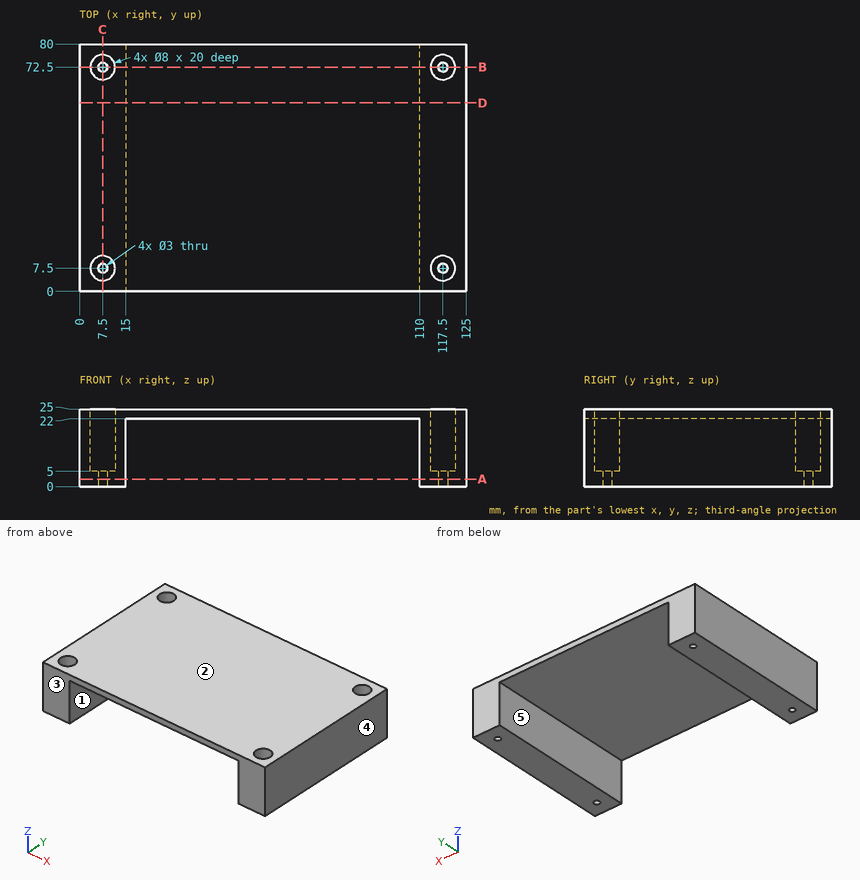
The figure shows three views and two pictorial views of one solid part (mm, origin at its lowest corner). Answer the questions. A direction names the side the tool comes from. Give positions to 0.01 mm unless a question says otherwise; leave off trailing zeros. Write each loop counter-clockwise with the first axis right and the second up, starting at its lowest first coordinate (ties: lowest second). Pieces come first, ordered by that corner, then holes. Notation, with made-up numbers: (73.25, 23.5) -> (119.25, 23.5) arc R30 ccw to (119.25, 53.5) -> close; hole circle Ø2 at (6.25, 82.25). An arc over 180 degrees is marked (long way). Write each question's results on one line, items separated by ' | '.
1. A tool of negligible diameter and unlimited length cuts with its end or side. For the marked faces 1 and 2, from which of +Z, -Z, +X, -X, +Y, -Y can it reach the whole face along a straight path? Write none if from no direction.
Data:
face 1: -Z, +Y, -Y | face 2: +Z, +X, -X, +Y, -Y
2. Find section D-D on y = 61. Determine the outline of the cut face in (x, z).
Data:
outline: (0, 0) -> (15, 0) -> (15, 22) -> (110, 22) -> (110, 0) -> (125, 0) -> (125, 25) -> (0, 25) -> close
3. Find section C-C on x = 7.5. Determine the outline of the cut face in (y, z), and give its area (3 significant figures).
Data:
outline: (0, 0) -> (6, 0) -> (6, 5) -> (3.5, 5) -> (3.5, 25) -> (0, 25) -> close; (9, 0) -> (71, 0) -> (71, 5) -> (68.5, 5) -> (68.5, 25) -> (11.5, 25) -> (11.5, 5) -> (9, 5) -> close; (74, 0) -> (80, 0) -> (80, 25) -> (76.5, 25) -> (76.5, 5) -> (74, 5) -> close | area: 1,650 mm^2
4. Find section B-B on y = 72.5. Determine the outline of the cut face in (x, z), and give its area (3 significant figures).
Data:
outline: (0, 0) -> (6, 0) -> (6, 5) -> (3.5, 5) -> (3.5, 25) -> (0, 25) -> close; (9, 0) -> (15, 0) -> (15, 22) -> (110, 22) -> (110, 0) -> (116, 0) -> (116, 5) -> (113.5, 5) -> (113.5, 25) -> (11.5, 25) -> (11.5, 5) -> (9, 5) -> close; (119, 0) -> (125, 0) -> (125, 25) -> (121.5, 25) -> (121.5, 5) -> (119, 5) -> close | area: 685 mm^2
5. Each of these flat-tipped pins is pushed along its axis until it touches: pin 1 Ø6.5 at (x, y) = (117.5, 71.5) entering from +Z; pin 2 Ø4 at (x, y) = (117, 7) entering from +Z. Where does it stop, or does it pass through?
Data:
pin 1: z = 25 | pin 2: z = 5
6. Determine the mould class of the marked faces 3, 4 and 5 for opening direction X: +X half, -X half, draft (parallel to the pull), parting line (faces both ways), or undercut.
Data:
face 3: draft | face 4: +X half | face 5: undercut
7. Find section A-A on z = 2.5. Determine the outline of the cut face in (x, y).
Data:
outline: (0, 0) -> (15, 0) -> (15, 80) -> (0, 80) -> close; (110, 0) -> (125, 0) -> (125, 80) -> (110, 80) -> close; hole circle Ø3 at (7.5, 7.5); hole circle Ø3 at (7.5, 72.5); hole circle Ø3 at (117.5, 7.5); hole circle Ø3 at (117.5, 72.5)
8. Straight lines are drawn through the part: L1, parallel to Y at x = 7.5, z = 2.3; L2, parallel to Y at x = 117.5, z = 19; L3, parallel to X at y = 57.5, z = 18.75. For each, find the intervals that lie inside material, in ascending order.
Data:
L1: 0 to 6, 9 to 71, 74 to 80 | L2: 0 to 3.5, 11.5 to 68.5, 76.5 to 80 | L3: 0 to 15, 110 to 125
